from build123d import *
from build123d.topology import SkipClean

# Parameters (mm, degrees)
SKETCH1_W           = 38.452994616
SKETCH1_H           = 5
BOSS_EXTRUDE1_DEPTH = 75
BOSS_EXTRUDE2_DEPTH = 10
BOSS_EXTRUDE4_DEPTH = 75
BOSS_EXTRUDE5_START = -65
BOSS_EXTRUDE5_DEPTH = 10
CUT_EXTRUDE7_START  = -10
CUT_EXTRUDE7_DEPTH  = 55
SKETCH5_R           = 3.175
CUT_EXTRUDE8_DEPTH  = 55


with BuildPart() as part:
    # Sketch1 → Boss-Extrude1 (new body)
    with BuildSketch(Plane.XY):
        with Locations((25, -2.5)):
            Rectangle(SKETCH1_W, SKETCH1_H)
    extrude(amount=-BOSS_EXTRUDE1_DEPTH)

    # Sketch1_4 → Boss-Extrude2 (add)
    with BuildSketch(Plane.XY):
        with BuildLine():
            ThreePointArc((10.773502692, -5), (9.309036598, -1.464466094), (5.773502692, 0))
            Line((5.773502692, 0), (5.773502692, -2.5))
            ThreePointArc((5.773502692, -2.5), (7.541269645, -3.232233047), (8.273502692, -5))
            Line((8.273502692, -5), (10.773502692, -5))
        make_face()
        with BuildLine():
            Line((5.773502692, -2.5), (5.773502692, 0))
            ThreePointArc((5.773502692, 0), (3.273502704, -0.669872974), (1.443375686, -2.499999977))
            ThreePointArc((1.443375686, -2.499999977), (4.479407453, -9.829629128), (10.773502692, -5))
            Line((10.773502692, -5), (8.273502692, -5))
            ThreePointArc((8.273502692, -5), (4.005735739, -6.767766953), (5.773502692, -2.5))
        make_face()
        with BuildLine():
            ThreePointArc((8.273502692, -5), (7.541269645, -3.232233047), (5.773502692, -2.5))
            Line((5.773502692, -2.5), (5.773502692, -5))
            Line((5.773502692, -5), (8.273502692, -5))
        make_face()
        with BuildLine():
            Line((5.773502692, -5), (5.773502692, -2.5))
            ThreePointArc((5.773502692, -2.5), (4.005735739, -6.767766953), (8.273502692, -5))
            Line((8.273502692, -5), (5.773502692, -5))
        make_face()
    extrude(amount=-BOSS_EXTRUDE2_DEPTH)

    # Sketch1_11 → Boss-Extrude4 (add)
    with BuildSketch(Plane.XY):
        with BuildLine():
            ThreePointArc((8.273502692, -5), (7.541269645, -3.232233047), (5.773502692, -2.5))
            Line((5.773502692, -2.5), (5.773502692, -5))
            Line((5.773502692, -5), (8.273502692, -5))
        make_face()
        with BuildLine():
            Line((5.773502692, -5), (5.773502692, -2.5))
            ThreePointArc((5.773502692, -2.5), (4.005735739, -6.767766953), (8.273502692, -5))
            Line((8.273502692, -5), (5.773502692, -5))
        make_face()
    extrude(amount=-BOSS_EXTRUDE4_DEPTH)

    # Sketch1_12 → Boss-Extrude5 (add)
    with BuildSketch(Plane.XY.offset(BOSS_EXTRUDE5_START)):
        with BuildLine():
            ThreePointArc((10.773502692, -5), (9.309036598, -1.464466094), (5.773502692, 0))
            Line((5.773502692, 0), (5.773502692, -2.5))
            ThreePointArc((5.773502692, -2.5), (7.541269645, -3.232233047), (8.273502692, -5))
            Line((8.273502692, -5), (10.773502692, -5))
        make_face()
        with BuildLine():
            Line((5.773502692, -2.5), (5.773502692, 0))
            ThreePointArc((5.773502692, 0), (3.273502704, -0.669872974), (1.443375686, -2.499999977))
            ThreePointArc((1.443375686, -2.499999977), (4.479407453, -9.829629128), (10.773502692, -5))
            Line((10.773502692, -5), (8.273502692, -5))
            ThreePointArc((8.273502692, -5), (4.005735739, -6.767766953), (5.773502692, -2.5))
        make_face()
    extrude(amount=-BOSS_EXTRUDE5_DEPTH)

    # Sketch1_13 → Cut-Extrude7 (cut)
    with SkipClean():  # the faces are left unmerged after this step: merging them gives an invalid solid
        with BuildSketch(Plane.XY.offset(CUT_EXTRUDE7_START)):
            with BuildLine():
                ThreePointArc((10.773502692, -5), (9.309036598, -1.464466094), (5.773502692, 0))
                Line((5.773502692, 0), (5.773502692, -2.5))
                ThreePointArc((5.773502692, -2.5), (7.541269645, -3.232233047), (8.273502692, -5))
                Line((8.273502692, -5), (10.773502692, -5))
            make_face()
            with BuildLine():
                Line((5.773502692, -2.5), (5.773502692, 0))
                ThreePointArc((5.773502692, 0), (3.273502704, -0.669872974), (1.443375686, -2.499999977))
                ThreePointArc((1.443375686, -2.499999977), (4.479407453, -9.829629128), (10.773502692, -5))
                Line((10.773502692, -5), (8.273502692, -5))
                ThreePointArc((8.273502692, -5), (4.005735739, -6.767766953), (5.773502692, -2.5))
            make_face()
        extrude(amount=-CUT_EXTRUDE7_DEPTH, mode=Mode.SUBTRACT)

    # Sketch5 → Cut-Extrude8 (cut)
    with SkipClean():  # the faces are left unmerged after this step: merging them gives an invalid solid
        with BuildSketch(Plane.XZ.offset(5)):
            with Locations((25, -25)):
                Circle(SKETCH5_R)
            with Locations((25, -50)):
                Circle(SKETCH5_R)
        extrude(amount=-CUT_EXTRUDE8_DEPTH, mode=Mode.SUBTRACT)


solid = part.part
Check sheet for the modelled part. Datum: model origin and axes. Units: mm. A direction names the side the tool comes from. Round coordinates to 2 decimals unless told otherwise and drop trailing zeros. Write each loop counter-clockwise with the first axis right and the second up, starting at its lowest first coordinate (ties: lowest second). Pieces come first, ordered by that corner, then holes. Notation, with made-up numbers: (26.25, -37) -> (65.25, -37) arc R13 ccw to (65.25, -20) -> close; hole circle Ø3 at (38.5, -40). An arc over 180 degrees is marked (long way). Answer as CSV lines item,"result". Start each with the question number.
1) Release check for a two-part mould opening along X. For faces 1 (the cylindrical face through (24.31, -2.54, -53.1)), 2 (the flat face through (22, -4, -75)), 3 (the flat face through (44.226, -3, -37)) record: pulls with the +X half, pulls with the -X half, needs draft (parallel to the pull), parting line crosses it, or undercut.
2) Section check A-A on x = 25. Enter the section's corners in (y, z) (3 decimals).
3) Section check B-B on z = -50. Enter the section's corners in (x, y) (1 decimal).
4) Material ranges on line 1 (Z direction, x = 25, y = -3.65) (3 decimals); line 2 (X direction, y = -4.75, z = -58.5); line 3 (X direction, y = -3.5, z = -52.5), recorded low to high. Write a range as from..to.
5) Section check C-C on z = -32. Enter the section's corners in (x, y), and give its area (3 significant figures).
6) Go/stop test with a flat-tipped pin: P1, Ø10, axis at x = 25, z = -25, coming from the -Y side. Record where the tip stops, or that it passes through.
7) Tool access check on faces 4 (the flat face through (22, -4, 0)), 5 (the flat face through (27, -5, -37)), 6 (the cylindrical face through (9.348, -1.504, -37.115)). Record the directions out of +Z, -Z, +X, -X, +Y, -Y that give a thin tool (end or side, any length) a straight path to the whole face; none if there is none.
8) Section check D-D on y = -8.25. Enter the section's corners in (x, z), and give its area (3 significant figures).
Found:
1,face 1,"undercut"
1,face 2,"needs draft"
1,face 3,"pulls with the +X half"
2,outline,"(-5, -75) -> (0, -75) -> (0, -53.175) -> (-5, -53.175) -> close; (-5, -46.825) -> (0, -46.825) -> (0, -28.175) -> (-5, -28.175) -> close; (-5, -21.825) -> (0, -21.825) -> (0, 0) -> (-5, 0) -> close"
3,outline,"circle Ø5 at (5.8, -5); (5.8, 0) arc R5 cw to (10.8, -5) -> (21.8, -5) -> (21.8, 0) -> close; (28.2, -5) -> (44.2, -5) -> (44.2, 0) -> (28.2, 0) -> close"
4,line 1,"z = -75..-53.175, -46.825..-28.175, -21.825..0"
4,line 2,"x = 3.29..8.26, 10.77..44.23"
4,line 3,"x = 3.77..7.77, 10.54..23.04, 26.96..44.23"
5,outline,"circle Ø5 at (5.77, -5); (5.77, 0) arc R5 cw to (10.77, -5) -> (44.23, -5) -> (44.23, 0) -> close"
5,area,"192 mm^2"
6,P1,"stops at y = -5"
7,face 4,"+Z, +X, -X, +Y, -Y"
7,face 5,"+Z, -Z, +X, -Y"
7,face 6,"none"
8,outline,"(1.97, -75) -> (9.57, -75) -> (9.57, -65) -> (1.97, -65) -> close; (1.97, -10) -> (9.57, -10) -> (9.57, 0) -> (1.97, 0) -> close"
8,area,"152 mm^2"
